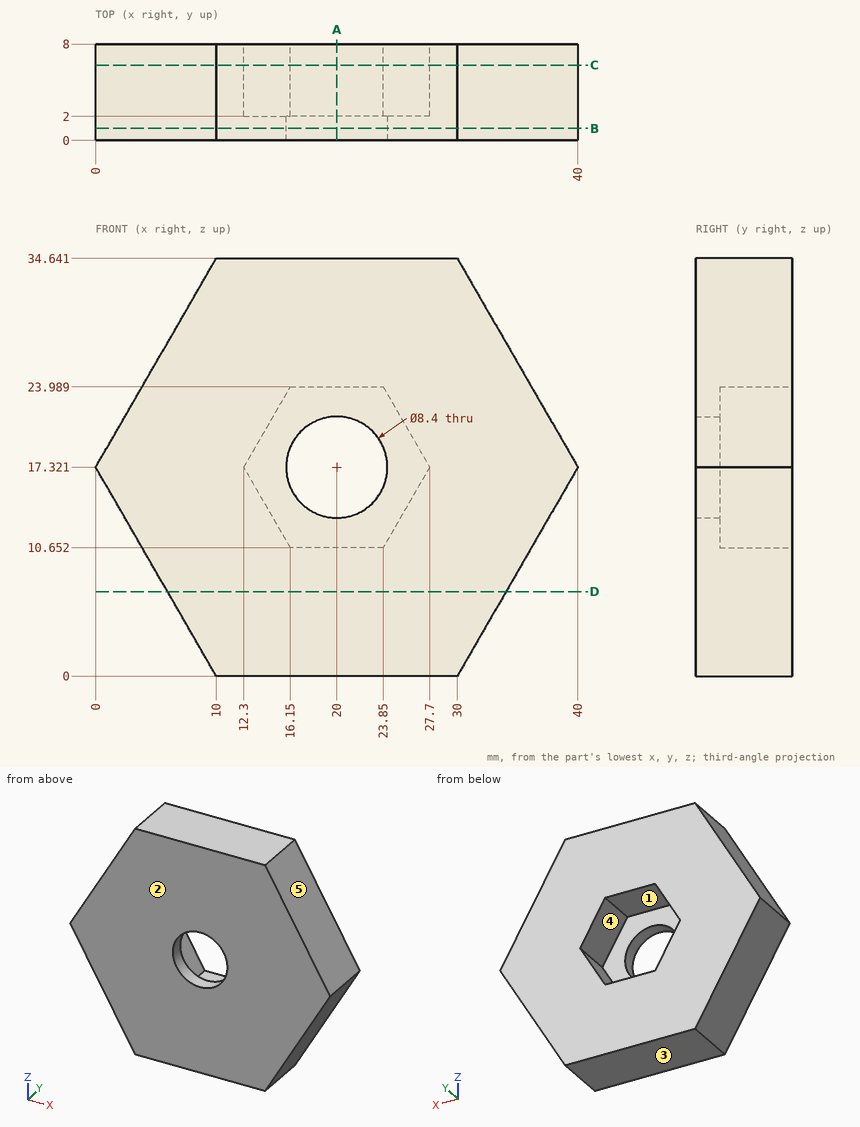
Geometry: see drawing. Coordinates: mm, zero at the bounding-box minimum. A direction names the side the tool comes from. Give positions to 0.01 mm unless a question says otherwise; leave off trailing zeros. Order: outer loops, then holes, each group sorted by start corner. A loop starts at its lowest first (then second) coordinate and runs counter-clockwise, first axis right, second up. Notation, with made-up numbers: M -37.5,50.5 L -16.5,50.5 A31 cw -16.5,75.5 Z; hole C -29.75,-17 d9. An arc over 180 degrees is marked long. Answer as CSV lines item,"result". Start each with the question number.
1) Cut plane A-A (x = 20). Output: boundary loops of the cut face in (y, z).
2) Cut plane D-D (z = 7). Output: boundary loops of the cut face in (x, y).
3) Cut plane B-B (y = 1). Output: boundary loops of the cut face in (x, z), then the cut area to 3 significant figures.
4) Line query: line 1 (Z direction, x = 20, y = 1.55); line 2 (Z direction, x = 18.5, y = 3); line 3 (X direction, y = 5.5, z = 23). Output: solid intervals per line, ascending. Write a range as from..to.
5) Set-up query: the marked faces 4 and 5. Return all of +Z, -Z, +X, -X, +Y, -Y with unobstructed straight access to the full face (end or side cutting, diameter ignored); none if empty.
6) Mould query, pull axis Z, two halves, no side actions, for the marked faces 1, 2 and 3. Classes: +Z half, -Z half, draft (parallel to the pull), parting line (faces both ways), or undercut.
7) First-contact query: P1, Ø6.5, axis at x = 21.5, z = 16, coming from the +Y side; P2, Ø1.5, axis at y = 5.5, z = 29, coming from the -X side; P3, Ø3, axis at y = 4.5, z = 4, coming from the -X side (1 decimal). Flat tips, straight axial feed; report the tip coordinate or a pass-through.
8) Cut plane C-C (y = 6.25). Output: boundary loops of the cut face in (x, z).
Findings below:
1,outline,"M 0,0 L 8,0 L 8,10.65 L 2,10.65 L 2,13.12 L 0,13.12 Z; M 0,21.52 L 2,21.52 L 2,23.99 L 8,23.99 L 8,34.64 L 0,34.64 Z"
2,outline,"M 5.96,0 L 34.04,0 L 34.04,8 L 5.96,8 Z"
3,outline,"M 0,17.32 L 10,0 L 30,0 L 40,17.32 L 30,34.64 L 10,34.64 Z; hole C 20,17.32 d8.4"
3,area,"984 mm²"
4,line 1,"z = 0..13.12, 21.52..34.64"
4,line 2,"z = 0..10.65, 23.99..34.64"
4,line 3,"x = 3.28..15.58, 24.42..36.72"
5,face 4,"+Y"
5,face 5,"+Z, +X, +Y, -Y"
6,face 1,"undercut"
6,face 2,"draft"
6,face 3,"-Z half"
7,P1,"stops at y = 2"
7,P2,"stops at x = 6.31"
7,P3,"stops at x = 6.8"
8,outline,"M 0,17.32 L 10,0 L 30,0 L 40,17.32 L 30,34.64 L 10,34.64 Z; hole M 12.3,17.32 L 16.15,10.65 L 23.85,10.65 L 27.7,17.32 L 23.85,23.99 L 16.15,23.99 Z"
